Geometry: final body of the model. Coordinates: model frame, mm. Face numbers are marked on the shaded views. A direction names the side the tool comes from. Round coordinates to 2 decimals unless told otherwise and drop trailing zeros. Write each loop counter-clockwise with the first axis right and the second up, starting at its lowest first coordinate (ties: lowest second). Pieces come first, ordered by that corner, then holes. Notation, with made-up numbers: (32, 65.5) -> (48, 65.5) arc R27 cw to (48, 83.5) -> close; hole circle Ø2 at (-34, 1.25). An arc over 180 degrees is marked (long way). Use one line per item in the form item = value. Start each with the question number.
1. Cut plane B-B, the plane y = 0. Return the cut outline in (x, z), plus the area to 3 significant figures.
2. Line query: L1, parallel to Y at x = -87, z = -8; L2, parallel to Y at x = 123.5, z = 54; L3, parallel to X at y = -0.5, z = -25. Output: solid intervals per line, ascending.
3. Cut plane D-D, the plane z = 35. Return the cut outline in (x, y), plus the area to 3 significant figures.
4. Cut plane A-A, the plane z = -31. Return the cut outline in (x, y).
5. Cut plane C-C, the plane x = -56.5. Return the cut outline in (y, z), plus the area to 3 significant figures.
6. Reachability of the marked faces 5, 6, 7 and 8 from +Z, -Z, +X, -X, +Y, -Y: full face, straight path, thin tool, end or side. Return the list, or none.
7. Pin query (flat end, axial travel): pin 1 Ø20 at (y, z) = (-86.5, -28.5) entering from +X; pin 2 Ø4 at (y, z) = (38.5, -17.5) entering from +X; pin 3 Ø6 at (y, z) = (-24, 45) entering from +X. Return the tip coordinate at first contact, or that it passes through.
8. Draft query along Y for the marked faces 1, 2, 3 and 4. Return one class per face: pulls with the +Y half, pulls with the -Y half, needs draft (parallel to the pull), parting line crosses it, or undercut.
```python
from build123d import *

# Parameters (mm, degrees)
RESSALTO_EXTRUS_O4_DEPTH = 20
RESSALTO_EXTRUS_O5_START = 40
ESBO_O6_R                = 50.5
RESSALTO_EXTRUS_O5_DEPTH = 40
RESSALTO_EXTRUS_O6_START = 40
RESSALTO_EXTRUS_O6_DEPTH = 40
RESSALTO_EXTRUS_O7_START = 40
RESSALTO_EXTRUS_O7_DEPTH = 40
RESSALTO_EXTRUS_O8_START = 40
RESSALTO_EXTRUS_O8_DEPTH = 40
ESBO_O12_W               = 60
ESBO_O12_H               = 65.5
RESSALTO_EXTRUS_O9_DEPTH = 25


with BuildPart() as part:
    # Esboço2 → Ressalto-extrusão4 (new body)
    with BuildSketch(Plane.XY):
        with BuildLine():
            Line((-10, 115), (-10, 49.5))
            ThreePointArc((-10, 49.5), (-36.141814954, 35.270656526), (-49.729212576, 8.789506048))
            Line((-49.729212576, 8.789506048), (-115, 8.789506048))
            Line((-115, 8.789506048), (-115, -11.210493952))
            Line((-115, -11.210493952), (-49.239971825, -11.210493952))
            ThreePointArc((-49.239971825, -11.210493952), (-35.268472235, -36.143946467), (-10, -49.5))
            Line((-10, -49.5), (-10, -115))
            Line((-10, -115), (10, -115))
            Line((10, -115), (10, -49.5))
            Line((10, -49.5), (120, -31.5))
            ThreePointArc((120, -31.5), (151.5, 0), (120, 31.5))
            Line((120, 31.5), (10, 49.5))
            Line((10, 49.5), (10, 115))
            Line((10, 115), (-10, 115))
        make_face()
    extrude(amount=RESSALTO_EXTRUS_O4_DEPTH)

    # Esboço3 → Revolução2 (revolve)
    with BuildSketch(Plane(origin=(0, 0, 0), x_dir=(1, 0, 0), z_dir=(0, 1, 0)), mode=Mode.PRIVATE) as revolu_o2_sk:
        Polygon((120, -63), (120, -20), (151.5, -20), (142.5, -63), align=None)
    revolve(revolu_o2_sk.sketch.rotate(Axis((120, 0, 63), (0, 0, -1)), 90), axis=Axis((120, 0, 63), (0, 0, -1)))

    # Esboço5 → Corte-Revolução1 (revolve, cut)
    with BuildSketch(Plane(origin=(0, 0, 0), x_dir=(1, 0, 0), z_dir=(0, 1, 0)), mode=Mode.PRIVATE) as corte_revolu_o1_sk:
        Polygon((120, -20), (120, -63), (132.5, -63), (142.5, -20), align=None)
    revolve(corte_revolu_o1_sk.sketch.rotate(Axis((120, 0, 20), (0, 0, 1)), 180), axis=Axis((120, 0, 20), (0, 0, 1)), mode=Mode.SUBTRACT)

    # Esboço6 → Ressalto-extrusão5 (add)
    with BuildSketch(Plane(origin=(0, 0, 0), x_dir=(-1, 0, 0), z_dir=(0, 0, -1)).offset(RESSALTO_EXTRUS_O5_START)):
        Circle(ESBO_O6_R)
    extrude(amount=-RESSALTO_EXTRUS_O5_DEPTH)

    # Esboço7 → Ressalto-extrusão6 (add)
    with BuildSketch(Plane(origin=(0, 0, 0), x_dir=(-1, 0, 0), z_dir=(0, 0, -1)).offset(RESSALTO_EXTRUS_O6_START)):
        with BuildLine():
            Line((-10, -49.5), (-10, -115))
            Line((-10, -115), (10, -115))
            Line((10, -115), (10, -49.5))
            ThreePointArc((10, -49.5), (0, -50.5), (-10, -49.5))
        make_face()
    extrude(amount=-RESSALTO_EXTRUS_O6_DEPTH)

    # Esboço8 → Ressalto-extrusão7 (add)
    with BuildSketch(Plane(origin=(0, 0, 0), x_dir=(-1, 0, 0), z_dir=(0, 0, -1)).offset(RESSALTO_EXTRUS_O7_START)):
        with BuildLine():
            Line((10, 49.5), (10, 115))
            Line((10, 115), (-10, 115))
            Line((-10, 115), (-10, 49.5))
            ThreePointArc((-10, 49.5), (0, 50.5), (10, 49.5))
        make_face()
    extrude(amount=-RESSALTO_EXTRUS_O7_DEPTH)

    # Esboço10 → Ressalto-extrusão8 (add)
    with BuildSketch(Plane(origin=(0, 0, 0), x_dir=(-1, 0, 0), z_dir=(0, 0, -1)).offset(RESSALTO_EXTRUS_O8_START)):
        with BuildLine():
            Line((49.239971825, -11.210493952), (115, -11.210493952))
            Line((115, -11.210493952), (115, 8.789506048))
            Line((115, 8.789506048), (49.729212576, 8.789506048))
            ThreePointArc((49.729212576, 8.789506048), (50.484897398, -1.234963456), (49.239971825, -11.210493952))
        make_face()
    extrude(amount=-RESSALTO_EXTRUS_O8_DEPTH)

    # Esboço12 → Ressalto-extrusão9 (add)
    with BuildSketch(Plane(origin=(0, 0, -40), x_dir=(-1, 0, 0), z_dir=(0, 0, -1))):
        with Locations((0, 82.25)):
            Rectangle(ESBO_O12_W, ESBO_O12_H)
        with Locations((0, -82.25)):
            Rectangle(ESBO_O12_W, ESBO_O12_H)
    extrude(amount=-RESSALTO_EXTRUS_O9_DEPTH)


solid = part.part
```
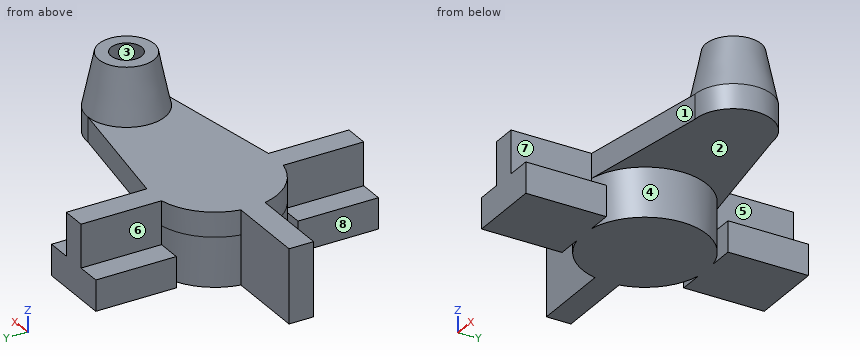
Outcome:
q1.outline = (-115, -40) -> (50.5, -40) -> (50.5, 0) -> (151.5, 0) -> (151.5, 20) -> (142.5, 63) -> (132.5, 63) -> (142.5, 20) -> (97.5, 20) -> (107.5, 63) -> (97.5, 63) -> (88.5, 20) -> (-115, 20) -> close
q1.area = 12,800 mm^2
q2.L1 = -11.21 to 8.79
q2.L2 = -24.13 to -14.17, 14.17 to 24.13
q2.L3 = -115 to 50.5
q3.outline = circle Ø56.72 at (120, 0); hole circle Ø38.02 at (120, 0)
q3.area = 1,390 mm^2
q4.outline = (-115, -11.21) -> (-49.24, -11.21) arc R50.5 ccw to (-10, -49.5) -> (-30, -49.5) -> (-30, -115) -> (30, -115) -> (30, -49.5) -> (10, -49.5) arc R50.5 ccw to (10, 49.5) -> (30, 49.5) -> (30, 115) -> (-30, 115) -> (-30, 49.5) -> (-10, 49.5) arc R50.5 ccw to (-49.73, 8.79) -> (-115, 8.79) -> close
q5.outline = (-11.21, -40) -> (8.79, -40) -> (8.79, 20) -> (-11.21, 20) -> close
q5.area = 1,200 mm^2
q6.face_5 = +Z, +X, +Y
q6.face_6 = +Z, -X, +Y
q6.face_7 = +Z, +X, -Y
q6.face_8 = +Z, -Z, -X, -Y
q7.pin_1 = 30
q7.pin_2 = 34.9
q7.pin_3 = 135.91
q8.face_1 = pulls with the -Y half
q8.face_2 = needs draft
q8.face_3 = undercut
q8.face_4 = undercut
